```python
from build123d import *

# Parameters (mm, degrees)
SKETCH1_W           = 90
SKETCH1_H           = 90
BOSS_EXTRUDE1_DEPTH = 30
SKETCH2_W           = 60
SKETCH2_H           = 60
BOSS_EXTRUDE2_DEPTH = 700
SKETCH3_R           = 10
CUT_EXTRUDE1_DEPTH  = 76
SKETCH4_R           = 15
BOSS_EXTRUDE3_DEPTH = 10


with BuildPart() as part:
    # Sketch1 → Boss-Extrude1 (new body)
    with BuildSketch(Plane(origin=(0, 0, 0), x_dir=(1, 0, 0), z_dir=(0, 1, 0))):
        Rectangle(SKETCH1_W, SKETCH1_H)
    extrude(amount=BOSS_EXTRUDE1_DEPTH)

    # Sketch2 → Boss-Extrude2 (add)
    with BuildSketch(Plane.XZ):
        Rectangle(SKETCH2_W, SKETCH2_H)
    extrude(amount=BOSS_EXTRUDE2_DEPTH)

    # Sketch3 → Cut-Extrude1 (cut, through all)
    with BuildSketch(Plane.XY.offset(30)):
        with Locations((2.6929442, -650)):
            Circle(SKETCH3_R)
    extrude(amount=-CUT_EXTRUDE1_DEPTH, mode=Mode.SUBTRACT)

    # Sketch4 → Boss-Extrude3 (add)
    with BuildSketch(Plane(origin=(0, 30, 0), x_dir=(1, 0, 0), z_dir=(0, 1, 0))):
        Circle(SKETCH4_R)
    extrude(amount=BOSS_EXTRUDE3_DEPTH)


solid = part.part
```
Check sheet for the modelled part. Datum: model origin and axes. Units: mm. A direction names the side the tool comes from. Round coordinates to 2 decimals unless told otherwise and drop trailing zeros. Write each loop counter-clockwise with the first axis right and the second up, starting at its lowest first coordinate (ties: lowest second). Pieces come first, ordered by that corner, then holes. Notation, with made-up numbers: (18, -22) -> (22, -22) arc R15 cw to (22, -2) -> close; hole circle Ø4 at (-31.5, 8). An arc over 180 degrees is marked (long way). One line per question, with ' | ' between items. Start each with the question number.
1. Sectioned sample at B-B, the plane z = 0. Record the cut outline in (x, y).
2. Set-up check for faces 1 (the face through (-14.985, 34.93, -0.66)), 2 (the face through (30, -345, 0)), 3 (the face through (-30, -345, 0)): record each of +Z, -Z, +X, -X, +Y, -Y from which the full face is reachable in a straight line by a thin tool's end or side.
3. Sectioned sample at C-C, the plane x = 22. Record the cut outline in (y, z), then the cut area to 3 significant figures.
4. Depth check by flat-ended pin: pin 1 (2 mm diameter, centred on x = -6, z = 26.5, fed in from +Y); pin 2 (6 mm diameter, centred on x = 20.5, z = -31.5, fed in from -Y); pin 3 (1 mm diameter, centred on y = -569.5, z = -17.5, fed in from +X); pin 4 (12 mm diameter, centred on y = -134, z = -25, fed in from -X). Enter the tip coordinate at first touch or a pass-through.
5. Release check for a two-part mould opening along Y. For faces 4 (the face through (0, 40, 0)), 5 (the face through (0, -345, -30)), 6 (the face through (1.391, -640.085, 0.42)) record: +Y half, -Y half, draft (parallel to the pull), parting line (faces both ways), or undercut.
6. Sectioned sample at A-A, the plane y = -650. Record the cut outline in (x, z).
7. Scan lines: line 1 along Y through (x, z) = (4, -28.5); line 2 along X through (y, z) = (-650, -7); line 3 along Y through (x, z) = (-21.5, 14). Record each from-to range of solid material in increasing order. Write a range as from..to.
8. Sectioned sample at D-D, the plane y = -290. Record the cut outline in (x, z).
Taken from the geometry:
1) outline: (-45, 0) -> (-30, 0) -> (-30, -700) -> (30, -700) -> (30, 0) -> (45, 0) -> (45, 30) -> (15, 30) -> (15, 40) -> (-15, 40) -> (-15, 30) -> (-45, 30) -> close; hole circle Ø20 at (2.69, -650)
2) face 1: +Y | face 2: +Z, -Z, +X, -Y | face 3: +Z, -Z, -X, -Y
3) outline: (-700, -30) -> (0, -30) -> (0, -45) -> (30, -45) -> (30, 45) -> (0, 45) -> (0, 30) -> (-700, 30) -> close | area: 44,700 mm^2
4) pin 1: stops at y = 30 | pin 2: stops at y = -700 | pin 3: stops at x = 30 | pin 4: stops at x = -30
5) face 4: +Y half | face 5: draft | face 6: undercut
6) outline: (-30, -30) -> (-7.31, -30) -> (-7.31, 30) -> (-30, 30) -> close; (12.69, -30) -> (30, -30) -> (30, 30) -> (12.69, 30) -> close
7) line 1: y = -700..-659.91, -640.09..30 | line 2: x = -30..-7.31, 12.69..30 | line 3: y = -700..30
8) outline: (-30, -30) -> (30, -30) -> (30, 30) -> (-30, 30) -> close
